Geometry: see drawing. Coordinates: mm, zero at the bounding-box minimum. A direction names the side the tool comes from. Give positions to 0.01 mm unless a question says otherwise; leave off trailing zeros. Loops run counter-clockwise (first coordinate to the right, second up) from the corner with the lowest first, then second, coordinate; pieces in that order, holes last. Notation, with made-up numbers: M 25.25,59 L 29.25,59 A27 cw 29.25,83 Z; hole C 14.25,25.5 d7. An arc over 180 degrees is marked long. Return JSON: item names as keys, results as strings. Group by question number.
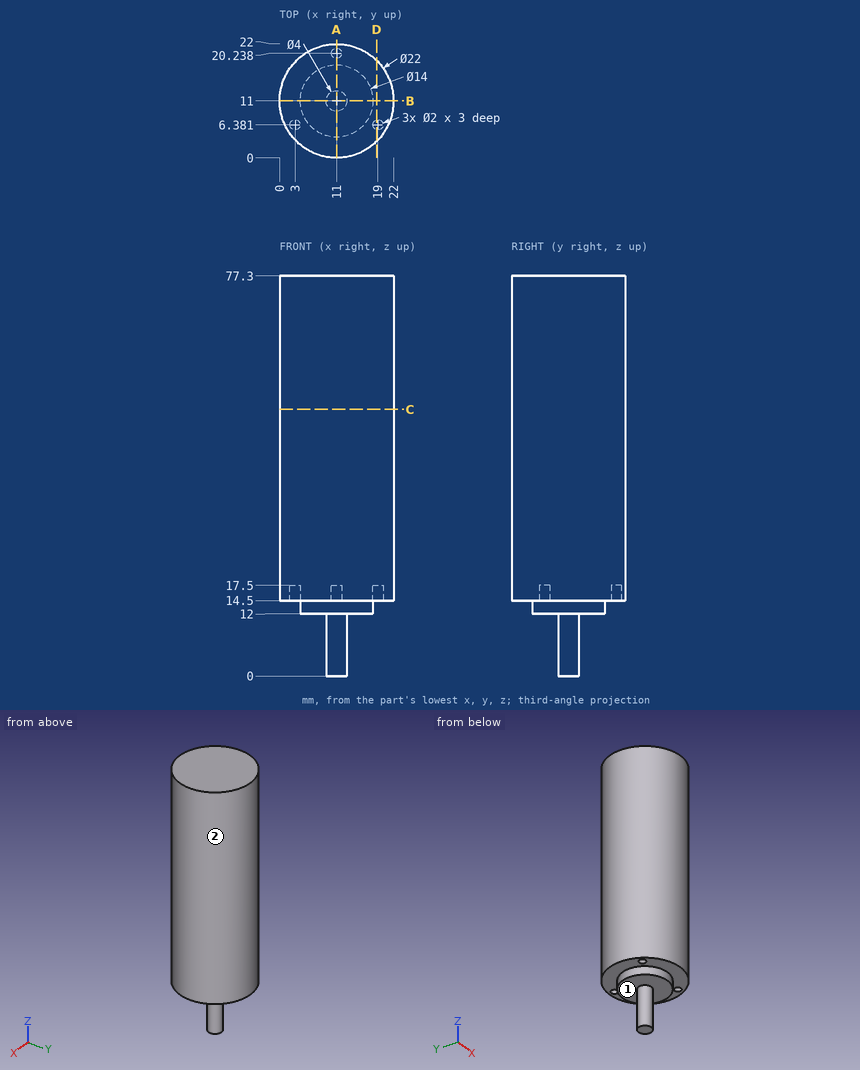
Item 1: Material intervals for line 1 (Y direction, x = 11, z = 15.35); line 2 (Z direction, x = 13.5, y = 13.25); line 3 (Y direction, x = 3, z = 16.1), sorted ascending. Write a range as from..to.
Item 2: Section A-A, the plane x = 11. Return loops of the section in (y, z), then the cut area to 3 significant figures.
Item 3: Section B-B, the plane y = 11. Return loops of the section in (x, z).
Item 4: Section D-D, the plane x = 18.75. Return loops of the section in (y, z), then the cut area to 3 significant figures.
Item 5: Reachability of the marked faces 1 and 2 from +Z, -Z, +X, -X, +Y, -Y: full face, straight path, thin tool, end or side. Return the list, or none.
Item 6: Section C-C, the plane z = 51.5. Return loops of the section in (x, y), then the cut area to 3 significant figures.
Item 7: First-contact query: pin 1 Ø6 at (y, z) = (17, 20) entering from -X; pin 2 Ø1 at (x, y) = (10.5, 20.5) entering from -Z; pin 3 Ø3 at (y, z) = (19, 21) entering from -X (1 decimal). Flat tips, straight axial feed; report the tip coordinate or a pass-through.
Answer below:
{
 "1": {"line 1": "0..19.24, 21.24..22", "line 2": "12..77.3", "line 3": "3.45..5.38, 7.38..18.55"},
 "2": {"outline": "M 0,14.5 L 4,14.5 L 4,12 L 9,12 L 9,0 L 13,0 L 13,12 L 18,12 L 18,14.5 L 19.24,14.5 L 19.24,17.5 L 21.24,17.5 L 21.24,14.5 L 22,14.5 L 22,77.3 L 0,77.3 Z", "area": "1,460 mm^2"},
 "3": {"outline": "M 0,14.5 L 4,14.5 L 4,12 L 9,12 L 9,0 L 13,0 L 13,12 L 18,12 L 18,14.5 L 22,14.5 L 22,77.3 L 0,77.3 Z"},
 "4": {"outline": "M 3.19,14.5 L 5.41,14.5 L 5.41,17.5 L 7.35,17.5 L 7.35,14.5 L 18.81,14.5 L 18.81,77.3 L 3.19,77.3 Z", "area": "975 mm^2"},
 "5": {"face 1": "-Z", "face 2": "+Z, -Z"},
 "6": {"outline": "C 11,11 d22", "area": "380 mm^2"},
 "7": {"pin 1": "x = 0.42", "pin 2": "z = 14.5", "pin 3": "x = 2.1"}
}
